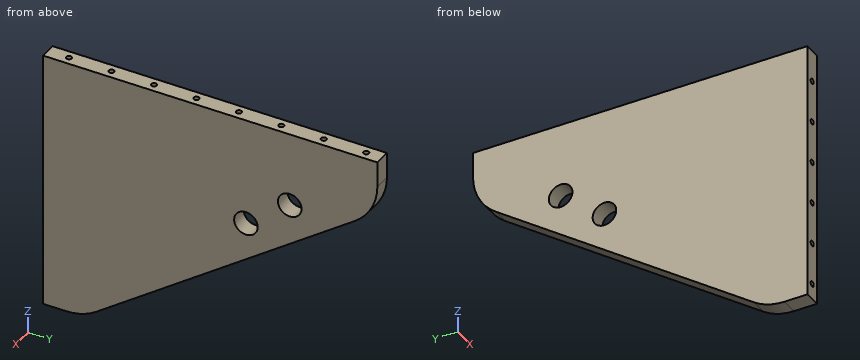
from build123d import *

# Parameters (mm, degrees)
BOSS_EXTRUDE1_DEPTH = 31.75
CUT_EXTRUDE1_DEPTH  = 813.777990905
LPATTERN1_COUNT     = 8
LPATTERN1_PITCH     = 80
LPATTERN2_COUNT     = 6
LPATTERN2_PITCH     = 80
SKETCH8_R           = 22.225
CUT_EXTRUDE2_DEPTH  = 813.777990905


with BuildPart() as part:
    # Sketch1 → Boss-Extrude1 (new body)
    with BuildSketch(Plane(origin=(0, 0, 0), x_dir=(0, 0, -1), z_dir=(1, 0, 0))):
        with BuildLine():
            Line((0, 0), (0, 640))
            Line((0, 640), (58.049523734, 640))
            ThreePointArc((58.049523734, 640), (104.150200697, 628.73966184), (139.86869342, 597.494551671))
            Line((139.86869342, 597.494551671), (481.819169686, 110.872720062))
            ThreePointArc((481.819169686, 110.872720062), (495.346517945, 83.528483741), (500, 53.378168391))
            Line((500, 53.378168391), (500, 0))
            Line((500, 0), (0, 0))
        make_face()
    extrude(amount=BOSS_EXTRUDE1_DEPTH)

    # Sketch2 → Cut-Extrude1 (cut, through all)
    with BuildSketch(Plane.ZY):
        Polygon((0, 640), (-10, 640), (-10, 10), (-500, 10), (-500, 0), (0, 0), align=None)
    extrude(amount=-CUT_EXTRUDE1_DEPTH, mode=Mode.SUBTRACT)

    # Sketch4 → M12 Tapped Hole1 (revolve, cut)
    with BuildSketch(Plane(origin=(15.875, 50, -10), x_dir=(0, -1, 0), z_dir=(1, 0, 0))):
        Polygon((0, 0), (0, 47.054389157), (5.1, 43.99), (5.1, 0), align=None)
    m12_tapped_hole1 = revolve(axis=Axis((15.875, 50, -3.65), (0, 0, -1)), mode=Mode.SUBTRACT)

    # LPattern1: M12 Tapped Hole1 ×8
    with Locations(*[(0, i * LPATTERN1_PITCH, 0) for i in range(1, LPATTERN1_COUNT)]):
        add(m12_tapped_hole1, mode=Mode.SUBTRACT)

    # Sketch6 → M12 Tapped Hole2 (revolve, cut)
    with BuildSketch(Plane(origin=(15.875, 10, -70), x_dir=(0, 0, -1), z_dir=(1, 0, 0))):
        Polygon((0, 0), (0, 47.054389157), (5.1, 43.99), (5.1, 0), align=None)
    m12_tapped_hole2 = revolve(axis=Axis((15.875, 3.65, -70), (0, 1, 0)), mode=Mode.SUBTRACT)

    # LPattern2: M12 Tapped Hole2 ×6
    with Locations(*[(0, 0, -i * LPATTERN2_PITCH) for i in range(1, LPATTERN2_COUNT)]):
        add(m12_tapped_hole2, mode=Mode.SUBTRACT)

    # Sketch8 → Cut-Extrude2 (cut, through all)
    with BuildSketch(Plane.ZY):
        with Locations((-213.2, 392.35)):
            Circle(SKETCH8_R)
        with Locations((-149.7, 474.9)):
            Circle(SKETCH8_R)
    extrude(amount=-CUT_EXTRUDE2_DEPTH, mode=Mode.SUBTRACT)


solid = part.part
Design review of the part built by this model. Coordinates are the model's own, in mm. Give positions to 0.01 mm unless a question says otherwise; leave off trailing zeros. Order: outer loops, then holes, each group sorted by start corner. A loop starts at its lowest first (then second) coordinate and runs counter-clockwise, first axis right, second up. Notation, with made-up numbers: (63, 6.5) - (114, 6.5) arc R4 cw to (114, 11.5) - close; hole circle Ø8 at (-19, -32). An arc over 180 degrees is marked (long way). Write item = value, one per line. Start each with the question number.
Q1. We need section C-C on z = -269.5. State the section outline as (x, y) points, plus the area to 3 significant figures.
Q2. We need section A-A on z = -201.5. State the section outline as (x, y) points.
Q3. We need section B-B on y = 556. State the section outline as (x, z) points, plus the area to 3 significant figures.
Q4. Clearance check with flat-ended pins moving along their axes: pin 1 Ø6 at (x, z) = (15.875, -70) entering from +Y; pin 2 Ø6 at (x, z) = (21, -94.5) entering from +Y; pin 3 Ø1.5 at (x, z) = (26, -180.5) entering from +Y. State where each tip first meets the part, or that it passes through.
Q5. To check wall thickness, follow L1, parallel to X at y = 130, z = -26 (3 decimals); L2, parallel to Z at x = 13, y = 458.5; L3, parallel to Z at x = 28.5, y = 468. State the ranges of each line that lie inside material, in increasing order. Write a range as from..to.
Working result:
q1.outline = (0, 10) - (31.75, 10) - (31.75, 413.02) - (0, 413.02) - close
q1.area = 12,800 mm²
q2.outline = (0, 10) - (31.75, 10) - (31.75, 373.45) - (0, 373.45) - close; (0, 411.25) - (31.75, 411.25) - (31.75, 509.79) - (0, 509.79) - close
q3.outline = (0, -169.03) - (31.75, -169.03) - (31.75, -10) - (0, -10) - close
q3.area = 5,050 mm²
q4.pin_1 = 639.6
q4.pin_2 = 634.24
q4.pin_3 = 540.74
q5.L1 = 0..10.775, 20.975..31.75
q5.L2 = -237.54..-164.7, -134.7..-10
q5.L3 = -230.86..-170.83, -128.57..-10
